Autodesk Inventor part; units mm, degrees
ref_plane "Plano inicial" through (0, 0, 0) normal (0, 0, 1) x (1, 0, 0)
ref_plane "Plano final" through (0, 0, 120) normal (0, 0, 1) x (1, 0, 0)
ref_plane "Plano de trabalho4" through (0, -25, 0) normal (0, 0.7071, -0.7071) x (1, 0, 0)
ref_plane "Plano inicial" through (0, 0, 0) normal (0, 0, 1) x (1, 0, 0)
ref_plane "Plano final" through (0, 0, 120) normal (0, 0, 1) x (1, 0, 0)
sketch "Esboço" plane through (0, 0, 0) normal (0, 0, 1) x (1, 0, 0)
  line L0 (-15, -21) -> (-15, 21)
  line L1 (-11, 25) -> (11, 25)
  line L2 (15, 21) -> (15, -21)
  line L3 (11, -25) -> (-11, -25)
  arc A0 (-15, -21) -> (-11, -25) centre (-11, -21) ccw
  arc A1 (15, 21) -> (11, 25) centre (11, 21) ccw
  arc A2 (-11, 25) -> (-15, 21) centre (-11, 21) ccw
  arc A3 (11, -25) -> (15, -21) centre (11, -21) ccw
  arc A4 (-11, 23) -> (-13, 21) centre (-11, 21) ccw
  line L4 (-11, 23) -> (11, 23)
  arc A5 (13, 21) -> (11, 23) centre (11, 21) ccw
  line L5 (13, 21) -> (13, -21)
  arc A6 (11, -23) -> (13, -21) centre (11, -21) ccw
  line L6 (11, -23) -> (-11, -23)
  arc A7 (-13, -21) -> (-11, -23) centre (-11, -21) ccw
  line L7 (-13, -21) -> (-13, 21)
  line L8 (0, 36.1598) -> (0, -36.1598) construction
  line L9 (-22.1598, 0) -> (22.1598, 0) construction
  dimension "d7" = 4
  dimension "d9" = 30
  dimension "d11" = 50
  dimension "d12" = 2
  dimension "d15" = 15
  dimension "d16" = 25
extrude "Corpo" add sketch "Esboço" along normal up to surface (120 mm away) from surface at 0
sketch "Sketch3" plane through (0, 0, 0) normal (0, 0, 1) x (1, 0, 0)
  line L0 (0, 0) -> (10, 0)
ref_plane "Work Plane3" through (0, 0, 0) normal (0, -1, 0) x (1, 0, 0)
sketch "Sketch4" plane through (0, 0, 0) normal (0, -1, 0) x (1, 0, 0)
  line L0 (-2, 0) -> (12, 0)
  line L1 (-2, 120) -> (12, 120)
  dimension "d18" = 120
ref_plane "Plano de trabalho4" through (0, -25, 0) normal (0, 0.7071, -0.7071) x (1, 0, 0)
split "Dividir1" plane through (0, -25, 0) removes the side toward (0, 0.7071, -0.7071)
ref_plane "Plano de trabalho5" through (0, -25, 120) normal (0, 0.7071, 0.7071) x (1, 0, 0)
split "Dividir2" plane through (0, -25, 120) removes the side toward (0, 0.7071, 0.7071)
equation "\"d7\" = G_IR"
equation "\"d9\" = G_W"
equation "\"d11\" = G_H"
equation "\"d12\" = G_T"
equation "\"d15\" = 0.5 * d9"
equation "\"d16\" = 0.5 * d11"
equation "\"d3\" = G_L"
equation "\"G_W\" = 30"
equation "\"G_H\" = 50"
equation "\"G_T\" = 2"
equation "\"G_IR\" = 4"
equation "\"G_L\" = d18"
equation "\"G_OFFSET_START\" = 0"
equation "\"G_OFFSET_END\" = 0"
equation "\"d14\" = G_OFFSET_END + B_L"
equation "\"B_L\" = 120"
properties part number "ISO 4019 - 50x30x2 - 120" material "Aço, suave"
Read the model definition and answer for the solid it produces. Units are mm, in the model's axes. A direction names the side the tool comes from. Round coordinates to 2 decimals unless told otherwise and drop trailing zeros. Order: outer loops, then holes, each group sorted by start corner. A loop starts at its lowest first (then second) coordinate and runs counter-clockwise, first axis right, second up. Notation, with made-up numbers: (84.5, -5) - (143.5, -5) arc R8 ccw to (143.5, 6) - close; hole circle Ø8 at (-15.75, -30.75). An arc over 180 degrees is marked (long way). Use one line per item in the form item = value. Start each with the question number.
(1) Find the intervals of material crossed by line 1 along X through (y, z) = (4.5, 90); line 2 along Y through (x, z) = (-7.5, 95); line 3 along X through (y, z) = (-22.5, 111), in increasing order. Write a range as from..to.
(2) The part is cut by section C-C (z = 55.5). Give the vertices of the cut face in (x, y), then the cut area to 3 significant figures.
(3) For faces 5 (the face through (-13, -5, 59)), 6 (the face through (13.797, 23.859, 59.804)), determine the directions among +Z, -Z, +X, -X, +Y, -Y from which every point of the face is accessible in a straight line to the end or side of a thin tool.
(4) Flat-ended cylindrical pins translate along their axes: pin 1 Ø4 at (x, z) = (-2, 42) entering from +Y; pin 2 Ø17.5 at (x, z) = (5.5, 31.5) entering from +Y; pin 3 Ø10 at (x, y) = (-9, -15) entering from +Z. Find the tip coordinate at first contact, or state that the pin passes through.
(5) Determine the mould class of faces 1 (the face through (-13.859, 23.797, 59.804)), 2 (the face through (13, -4, 59)), 3 (the face through (15, -4, 59)), 4 (the face through (0, 23, 60)) for opening direction Y: +Y half, -Y half, draft (parallel to the pull), parting line (faces both ways), or undercut.
(6) The part is cut by section A-A (y = -0.5). Give the vertices of the cut face in (x, z), then the cut area to 3 significant figures.
(7) The part is cut by section B-B (x = -2). Give the vertices of the cut face in (y, z), then the cut area to 3 significant figures.
Checked values:
q1.line_1 = -15..-13, 13..15
q1.line_2 = -25..-23
q1.line_3 = -14.71..-12.32, 12.32..14.71
q2.outline = (-15, -21) arc R4 ccw to (-11, -25) - (11, -25) arc R4 ccw to (15, -21) - (15, 21) arc R4 ccw to (11, 25) - (-11, 25) arc R4 ccw to (-15, 21) - close; hole (-13, -21) arc R2 ccw to (-11, -23) - (11, -23) arc R2 ccw to (13, -21) - (13, 21) arc R2 ccw to (11, 23) - (-11, 23) arc R2 ccw to (-13, 21) - close
q2.area = 294 mm^2
q3.face_5 = +Z, -Z
q3.face_6 = +Z, -Z, +X, +Y
q4.pin_1 = -23
q4.pin_2 = 11.01
q4.pin_3 = 113
q5.face_1 = +Y half
q5.face_2 = undercut
q5.face_3 = draft
q5.face_4 = undercut
q6.outline = (-15, 24.5) - (-13, 24.5) - (-13, 95.5) - (-15, 95.5) - close; (13, 24.5) - (15, 24.5) - (15, 95.5) - (13, 95.5) - close
q6.area = 284 mm^2
q7.outline = (-25, 0) - (-23, 2) - (-23, 118) - (-25, 120) - close; (23, 48) - (25, 50) - (25, 70) - (23, 72) - close
q7.area = 280 mm^2
